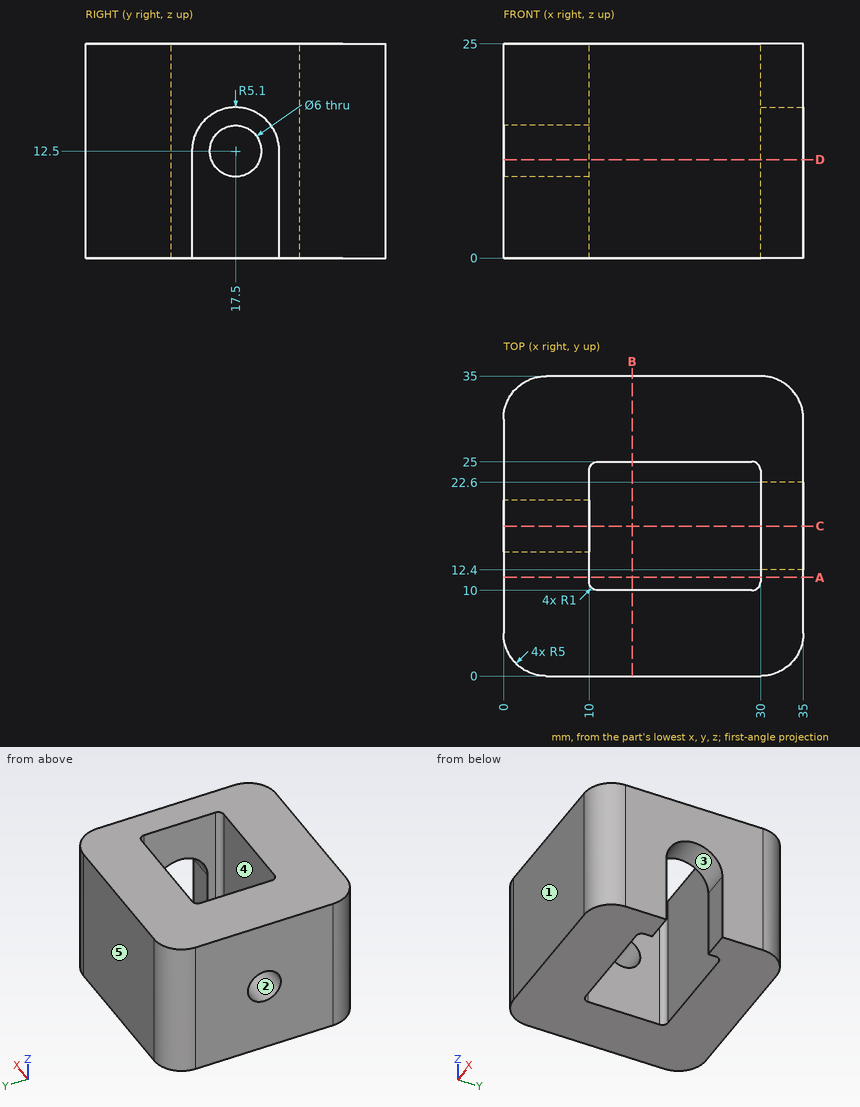
Check sheet for the drawn part. Datum: minimum x, y, z corner. Units: mm. A direction names the side the tool comes from. Round coordinates to 2 decimals unless told otherwise and drop trailing zeros. Loops run counter-clockwise (first coordinate to the right, second up) from the corner with the lowest first, then second, coordinate; pieces in that order, holes last. Notation, with made-up numbers: (63.5, 52.5) - (69.5, 52.5) arc R16 ccw to (69.5, 66.5) - close; hole circle Ø3 at (8, 14). An arc over 180 degrees is marked (long way). Answer as a JSON object with one key per item and string values. Group by question number.
Q1. Sectioned sample at C-C, the plane y = 17.5. Enter the section's corners in (x, z), plus the area to 3 significant figures.
Q2. Sectioned sample at B-B, the plane x = 15. Enter the section's corners in (y, z), plus the area to 3 significant figures.
Q3. Mould release check, pull along Z, two halves, no side actions. Record for the marked faces 1, 2 and 3: released by +Z, released by -Z, zero draft, split by the parting line, or undercut.
Q4. Scan lines: line 1 along Z through (x, y) = (4.75, 17.5); line 2 along Y through (x, z) = (17.5, 20.75); line 3 along X through (y, z) = (23, 23.5). Record each from-to range of solid material in increasing order. Write a range as [from, to].
Q5. Sectioned sample at D-D, the plane z = 11.5. Enter the section's corners in (x, y), plus the area to 3 significant figures.
Q6. Gauge pin test, flat ends, axial feed: P1, Ø2.5, axis at x = 32, z = 6, coming from the -Y side; P2, Ø7, axis at y = 17.5, z = 12.5, coming from the +X side; P3, Ø4, axis at x = 33.5, z = 7.5, coming from the +Y side. Record the tip position at first contact, or that the pin passes through.
Q7. Sectioned sample at A-A, the plane y = 11.5. Enter the section's corners in (x, z), plus the area to 3 significant figures.
Q8. Set-up check for the marked faces 4 and 5: record each of +Z, -Z, +X, -X, +Y, -Y from which the full face is reachable in a straight line by a thin tool's end or side.
Solution:
{
 "1": {"outline": "(0, 0) - (10, 0) - (10, 9.5) - (0, 9.5) - close; (0, 15.5) - (10, 15.5) - (10, 25) - (0, 25) - close; (30, 17.6) - (35, 17.6) - (35, 25) - (30, 25) - close", "area": "227 mm²"},
 "2": {"outline": "(0, 0) - (10, 0) - (10, 25) - (0, 25) - close; (25, 0) - (35, 0) - (35, 25) - (25, 25) - close", "area": "500 mm²"},
 "3": {"face 1": "zero draft", "face 2": "undercut", "face 3": "released by -Z"},
 "4": {"line 1": "z = [0, 9.5], [15.5, 25]", "line 2": "y = [0, 10], [25, 35]", "line 3": "x = [0, 10], [30, 35]"},
 "5": {"outline": "(0, 5) arc R5 ccw to (5, 0) - (30, 0) arc R5 ccw to (35, 5) - (35, 12.4) - (30, 12.4) - (30, 11) arc R1 cw to (29, 10) - (11, 10) arc R1 cw to (10, 11) - (10, 14.67) - (0, 14.67) - close; (0, 20.33) - (10, 20.33) - (10, 24) arc R1 cw to (11, 25) - (29, 25) arc R1 cw to (30, 24) - (30, 22.6) - (35, 22.6) - (35, 30) arc R5 ccw to (30, 35) - (5, 35) arc R5 ccw to (0, 30) - close", "area": "797 mm²"},
 "6": {"P1": "stops at y = 0.06", "P2": "stops at x = 10", "P3": "stops at y = 34.77"},
 "7": {"outline": "(0, 0) - (10, 0) - (10, 25) - (0, 25) - close; (30, 0) - (35, 0) - (35, 25) - (30, 25) - close", "area": "375 mm²"},
 "8": {"face 4": "+Z, -Z", "face 5": "+Z, -Z, +X, -X, +Y"}
}
